Check sheet for the modelled part. Datum: model origin and axes. Units: mm. Face numbers are marked on the shaded views. A direction names the side the tool comes from. Give positions to 0.01 mm unless a question says otherwise; leave off trailing zeros. Write each loop counter-clockwise with the first axis right and the second up, starting at its lowest first coordinate (ties: lowest second). Pieces come first, ordered by that corner, then holes. Notation, with made-up numbers: M -0.5,-16.75 L 40.5,-16.75 A22 ccw 40.5,11.25 Z; hole C -17,16.5 d4. An arc over 180 degrees is marked long. Write item = value, one per line. Start each with the question number.
1) Mould release check, pull along Y, two halves, no side actions. Record for the marked faces 1, 2, 3 and 4: released by +Y, released by -Y, zero draft, split by the parting line, or undercut.
2) Cross-section at C-C, the plane x = 7. Record the cut outline in (y, z).
3) Scan lines: line 1 along Z through (x, y) = (3, 86.5); line 2 along Y through (x, z) = (11.75, 32.5); line 3 along Y through (x, z) = (10.25, 15). Record each from-to range of solid material in increasing order. Write a range as [from, to].
4) Go/stop test with a flat-tipped pin: pin 1 (2 mm diameter, centred on x = 13.5, y = 107.5, fed in from +Z). Record where the tip stops, or that it passes through.
5) Cross-section at A-A, the plane z = 22. Record the cut outline in (x, y).
6) Access from +Z, -Z, +X, -X, +Y, -Y to the whole of each face (thin tool, end or side, straight path). Record for the marked faces 5 and 6.
7) Cross-section at B-B, the plane y = 85. Record the cut outline in (x, z).
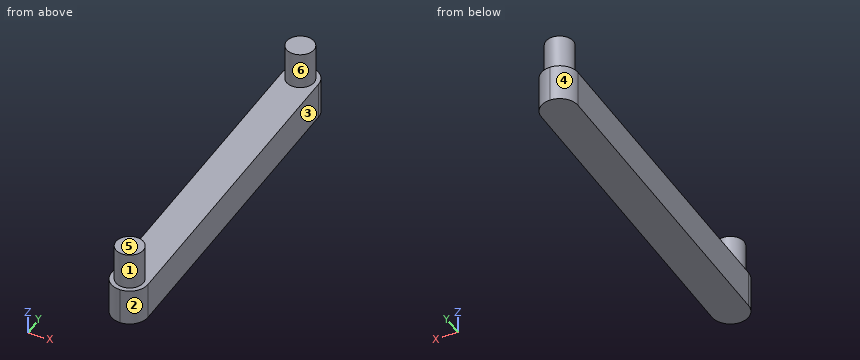
```python
from build123d import *

# Parameters (mm, degrees)
SKETCH1_W           = 20
SKETCH1_H           = 200
BOSS_EXTRUDE1_DEPTH = 20
FILLET1_R           = 10
FILLET2_R           = 10
FILLET3_R           = 10
FILLET4_R           = 10
SCALE1_SCALE        = 0.8
SKETCH2_R           = 6
BOSS_EXTRUDE3_DEPTH = 16


with BuildPart() as part:
    # Sketch1 → Boss-Extrude1 (new body)
    with BuildSketch(Plane.XY):
        with Locations((10, 100)):
            Rectangle(SKETCH1_W, SKETCH1_H)
    extrude(amount=BOSS_EXTRUDE1_DEPTH)

    # Fillet1
    fillet1_edges = [part.edges().sort_by_distance(p)[0] for p in [
        (20, 200, 10),
    ]]
    fillet(fillet1_edges, radius=FILLET1_R)

    # Fillet2
    fillet2_edges = [part.edges().sort_by_distance(p)[0] for p in [
        (0, 200, 10),
    ]]
    fillet(fillet2_edges, radius=FILLET2_R - 0.0001)  # a hair under: the kernel refuses the full size

    # Fillet3
    fillet3_edges = [part.edges().sort_by_distance(p)[0] for p in [
        (0, 0, 10),
    ]]
    fillet(fillet3_edges, radius=FILLET3_R)

    # Fillet4
    fillet4_edges = [part.edges().sort_by_distance(p)[0] for p in [
        (20, 0, 10),
    ]]
    fillet(fillet4_edges, radius=FILLET4_R - 0.0001)  # a hair under: the kernel refuses the full size


with BuildPart() as part_1:
    # Scale1: scaled about (10, 100, 10)
    add(part.part.scale(SCALE1_SCALE).moved(Location((2, 20, 2))))

    # Sketch2 → Boss-Extrude3 (add)
    with BuildSketch(Plane.XY.offset(18)):
        with Locations(Location((10, 172, 0), (0, 0, 180))):
            Circle(SKETCH2_R)
        with Locations(Location((10, 28, 0), (0, 0, 180))):
            Circle(SKETCH2_R)
    extrude(amount=BOSS_EXTRUDE3_DEPTH)


solid = part_1.part
```
Reply:
q1.face_1 = undercut
q1.face_2 = released by -Y
q1.face_3 = zero draft
q1.face_4 = released by +Y
q2.outline = M 20.58,2 L 179.42,2 L 179.42,18 L 177.2,18 L 177.2,34 L 166.8,34 L 166.8,18 L 33.2,18 L 33.2,34 L 22.8,34 L 22.8,18 L 20.58,18 Z
q3.line_1 = [2, 18]
q3.line_2 = [22.26, 33.74], [166.26, 177.74]
q3.line_3 = [20, 180]
q4.pin_1 = 18
q5.outline = C 10,28 d12; C 10,172 d12
q6.face_5 = +Z, +X, -X, +Y, -Y
q6.face_6 = +Z
q7.outline = M 2,2 L 18,2 L 18,18 L 2,18 Z
